Here's how the part is built. I have some questions about the finished solid (model axes, mm). A direction names the side the tool comes from. Give positions to 0.01 mm unless a question says otherwise; leave off trailing zeros. Loops run counter-clockwise (first coordinate to the right, second up) from the corner with the lowest first, then second, coordinate; pieces in that order, holes last.
Q1. I need wall thicknesses on probe 1 along X at (y, z) = (-3, 0.2); probe 2 along Y at (x, z) = (0.5, 0.4); probe 3 along Y at (x, z) = (-3, 0.1). Which ranges of each line are inside material? Lowest first, please.
Q2. For faces 1 (the face through (7.3, 0, 0.5)), 2 (the face through (16, -0.2, 0.5)), which set-ups out of +Z, -Z, +X, -X, +Y, -Y let a thin tool reach every point of the face, with its end or its side?
Q3. Suppose I cut it at A-A (x = 0). List the corners of the cut face in (y, z) for me.
Q4. Suppose I cut it at C-C (y = 2.5). List the corners of the cut face in (x, z) for me.
Q5. Thinking about a two-plate mould opening in Y: for faces 3 (the face through (0.1, 8, 0.5)), 4 (the face through (-0.2, 16, 0.5)), 5 (the face through (-7.3, 3.8, 1)), 6 (the face through (-0.2, -16, 0.5)), which applies, pulls with the +Y half, pulls with the -Y half, needs draft (parallel to the pull), parting line crosses it, or undercut?
Q6. Suppose I cut it at B-B (z = 0.3). List the corners of the cut face in (x, y) for me.
```python
from build123d import *

# Parameters (mm, degrees)
SKETCH_W     = 32
SKETCH_H     = 32
SKETCH_R     = 8
PAD_DEPTH    = 1
SKETCH001_W  = 2
SKETCH001_H  = 8
PAD001_DEPTH = 1


with BuildPart() as part:
    # Sketch → Pad (new body)
    with BuildSketch(Plane.XY):
        Rectangle(SKETCH_W, SKETCH_H)
        Circle(SKETCH_R, mode=Mode.SUBTRACT)
    extrude(amount=PAD_DEPTH)

    # Sketch001 (on Face7 of Pad) → Pad001 (join)
    with BuildSketch(Plane.XY.offset(1)):
        with Locations((-8.3, 0)):
            Rectangle(SKETCH001_W, SKETCH001_H)
        with Locations((8.3, 0)):
            Rectangle(SKETCH001_W, SKETCH001_H)
    extrude(amount=-PAD001_DEPTH)


solid = part.part
```
Solutions:
1. probe 1: x = -16 to -7.3, 7.3 to 16
1. probe 2: y = -16 to -7.98, 7.98 to 16
1. probe 3: y = -16 to -7.42, 7.42 to 16
2. face 1: +Z, -Z
2. face 2: +Z, -Z, +X, +Y, -Y
3. outline: (-16, 0) - (-8, 0) - (-8, 1) - (-16, 1) - close; (8, 0) - (16, 0) - (16, 1) - (8, 1) - close
4. outline: (-16, 0) - (-7.3, 0) - (-7.3, 1) - (-16, 1) - close; (7.3, 0) - (16, 0) - (16, 1) - (7.3, 1) - close
5. face 3: undercut
5. face 4: pulls with the +Y half
5. face 5: needs draft
5. face 6: pulls with the -Y half
6. outline: (-16, -16) - (16, -16) - (16, 16) - (-16, 16) - close; hole (-7.3, -3.27) arc R8 ccw to (7.3, -3.27) - (7.3, 3.27) arc R8 ccw to (-7.3, 3.27) - close
